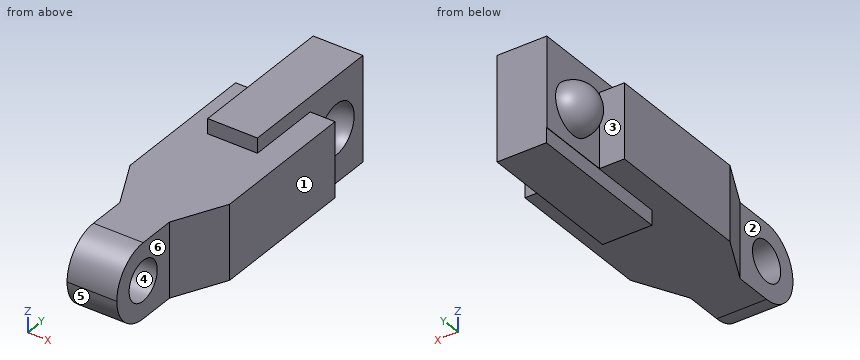
from build123d import *

# Parameters (mm, degrees)
SKETCH1_W            = 10
SKETCH1_H            = 30
BOSS_EXTRUDE1_DEPTH  = 15
BOSS_EXTRUDE5_DEPTH  = 15
SKETCH7_W            = 9.916734627
SKETCH7_H            = 30
BOSS_EXTRUDE7_DEPTH  = 3
SKETCH12_W           = 10
SKETCH12_H           = 15
BOSS_EXTRUDE9_DEPTH  = 15
SKETCH13_R           = 4
CUT_EXTRUDE3_DEPTH   = 15
FILLET2_R            = 7.5
SKETCH6_W            = 10
SKETCH6_H            = 30
BOSS_EXTRUDE11_DEPTH = 3


with BuildPart() as part:
    # Sketch1 → Boss-Extrude1 (new body)
    with BuildSketch(Plane.XY):
        with Locations((0.12195122, -8.922764228)):
            Rectangle(SKETCH1_W, SKETCH1_H)
    extrude(amount=BOSS_EXTRUDE1_DEPTH)

    # Sketch2 → Boss-Extrude5 (add)
    with BuildSketch(Plane.XY.offset(15)):
        Polygon((-4.87804878, -8.922764228), (-9.87804878, -8.922764228), (-9.87804878, -38.922764228), (-4.87804878, -48.922764228), (5.12195122, -48.922764228), (10.12195122, -38.922764228), (10.12195122, -8.922764228), (5.12195122, -8.922764228), (5.12195122, -23.922764228), (-4.87804878, -23.922764228), align=None)
    extrude(amount=-BOSS_EXTRUDE5_DEPTH)

    # Sketch7 → Boss-Extrude7 (add)
    with BuildSketch(Plane(origin=(0, 0, 0), x_dir=(-1, 0, 0), z_dir=(0, 0, -1))):
        with Locations((-0.163583906, -8.922764228)):
            Rectangle(SKETCH7_W, SKETCH7_H)
    extrude(amount=BOSS_EXTRUDE7_DEPTH)

    # Sketch12 → Boss-Extrude9 (add)
    with BuildSketch(Plane.XZ.offset(48.922764228)):
        with Locations((0.12195122, 7.5)):
            Rectangle(SKETCH12_W, SKETCH12_H)
    extrude(amount=BOSS_EXTRUDE9_DEPTH)

    # Sketch13 → Cut-Extrude3 (cut)
    with BuildSketch(Plane.ZY.offset(4.87804878)):
        with Locations((7.5, -56.422764228)):
            Circle(SKETCH13_R)
    extrude(amount=-CUT_EXTRUDE3_DEPTH, mode=Mode.SUBTRACT)

    # Fillet2
    fillet2_edges = [part.edges().sort_by_distance(p)[0] for p in [
        (0.12195122, -63.922764228, 0),
        (0.12195122, -63.922764228, 15),
    ]]
    fillet(fillet2_edges, radius=FILLET2_R - 0.0001)  # a hair under: the kernel refuses the full size

    # Sketch10 → Revolve3 (revolve)
    with BuildSketch(Plane.ZY.offset(4.87804878)):
        with BuildLine():
            Line((7.5, 3.577235772), (7.5, -6.422764228))
            ThreePointArc((7.5, -6.422764228), (2.5, -1.422764228), (7.5, 3.577235772))
        make_face()
    revolve(axis=Axis((-4.87804878, 3.577235772, 7.5), (0, -1, 0)))

    # Sketch15 → Cut-Revolve1 (revolve, cut)
    with BuildSketch(Plane(origin=(5.12195122, 0, 0), x_dir=(0, 0, -1), z_dir=(1, 0, 0))):
        with BuildLine():
            Line((-7.5, 3.577235772), (-7.5, -6.422764228))
            ThreePointArc((-7.5, -6.422764228), (-12.5, -1.422764228), (-7.5, 3.577235772))
        make_face()
    revolve(axis=Axis((5.12195122, 3.577235772, 7.5), (0, -1, 0)), mode=Mode.SUBTRACT)

    # Sketch6 → Boss-Extrude11 (add)
    with BuildSketch(Plane.XY.offset(15)):
        with Locations((0.12195122, -8.922764228)):
            Rectangle(SKETCH6_W, SKETCH6_H)
    extrude(amount=BOSS_EXTRUDE11_DEPTH)


solid = part.part
The listing builds one solid part. Answer for the finished solid, in the listing's coordinates (mm). Face numbers are marked on the shaded views. A direction names the side the tool comes from. Round coordinates to 2 decimals unless told otherwise and drop trailing zeros. Order: outer loops, then holes, each group sorted by start corner. A loop starts at its lowest first (then second) coordinate and runs counter-clockwise, first axis right, second up. Notation, with made-up numbers: M 70.25,87.25 L 106.25,87.25 A22 ccw 106.25,99.25 Z; hole C 79,-31.75 d1. An arc over 180 degrees is marked long. Answer in a Markdown table with one row per item. Add a question column.
1) Which of the six approach directions +Z, -Z, +X, -X, +Y, -Y give full straight-line access (tool end or side, diameter ignored) to the marked faces 1, 2 and 3?
2) Consider line 1 along Y through (x, z) = (-2.5, 7.5); line 2 along Y through (x, z) = (3.25, 7.5); line 3 along Y through (x, z) = (2.25, 7.5). Determine where each line is inside the solid, lowest interval first. Write a range as from..to.
3) Determine the mould class of the marked faces 4, 5 and 6 for opening direction Y: pulls with the +Y half, pulls with the -Y half, needs draft (parallel to the pull), parting line crosses it, or undercut.
4) The part is cut by section D-D on y = -4. Determine the outline of the cut face in (x, z), plus the area to 3 significant figures.
5) Flat-ended cylindrical pins translate along their axes: pin 1 Ø1 at (x, y) = (5.5, -45.5) entering from -Z; pin 2 Ø2.5 at (y, z) = (-15.5, -1.5) entering from -X; pin 3 Ø4 at (x, z) = (-7.5, 6.5) entering from +Y. Find the tip coordinate at first contact, or state that the pin passes through.
6) The part is cut by section A-A on x = 2.75. Count the separate pieces of the cut face and the enclosed holes in it, plus the area to 3 significant figures.
7) The part is cut by section B-B on y = -59. Determine the outline of the cut face in (x, z), plus the area to 3 significant figures.
8) The part is cut by section C-C on z = 13.25. Determine the outline of the cut face in (x, y), plus the area to 3 significant figures.
Findings below:
| question | item | result |
|---|---|---|
| 1 | face 1 | +Z, -Z, +X, +Y, -Y |
| 1 | face 2 | +Z, -Z, -X, -Y |
| 1 | face 3 | +Z, -Z, -X |
| 2 | line 1 | y = -63.92..-60.42, -52.42..6.08 |
| 2 | line 2 | y = -63.92..-60.42, -52.42..-6.06, 3.21..6.08 |
| 2 | line 3 | y = -63.92..-60.42, -52.42..-5.52, 2.67..6.08 |
| 3 | face 4 | undercut |
| 3 | face 5 | pulls with the -Y half |
| 3 | face 6 | needs draft |
| 4 | outline | M -4.88,0 L -4.79,0 L -4.79,-3 L 5.12,-3 L 5.12,3.22 A4.28 cw 5.12,11.78 L 5.12,18 L -4.88,18 L -4.88,11.78 A4.28 ccw -4.88,3.22 Z |
| 4 | area | 210 mm² |
| 5 | pin 1 | stops at z = 0 |
| 5 | pin 2 | stops at x = -4.79 |
| 5 | pin 3 | stops at y = 3.51 |
| 6 | separate pieces | 1 |
| 6 | enclosed holes | 2 |
| 6 | area | 1,090 mm² |
| 7 | outline | M -4.88,0.46 L 5.12,0.46 L 5.12,4.44 L -4.88,4.44 Z; M -4.88,10.56 L 5.12,10.56 L 5.12,14.54 L -4.88,14.54 Z |
| 7 | area | 79.7 mm² |
| 8 | outline | M -9.88,-38.92 L -4.88,-48.92 L -4.88,-61.24 L 5.12,-61.24 L 5.12,-48.92 L 10.12,-38.92 L 10.12,-8.92 L 5.12,-8.92 L 5.12,6.08 L -4.88,6.08 L -4.88,-8.92 L -9.88,-8.92 Z |
| 8 | area | 1,020 mm² |
